Input: dimensioned drawing with shaded views. Units: mm. Origin: part minimum x, y, z. A direction names the side the tool comes from. Give positions to 0.01 mm unless a question says otherwise; leave off trailing zeros. Write each loop counter-clockwise with the first axis right and the second up, starting at its lowest first coordinate (ties: lowest second). Pieces come first, ordered by that corner, then holes. Notation, with made-up numbers: M 4.25,33 L 25.25,33 A31 cw 25.25,66 Z; hole C 40.25,77 d10. An arc over 180 degrees is marked long. Answer as a JSON object with one key per item and string values.
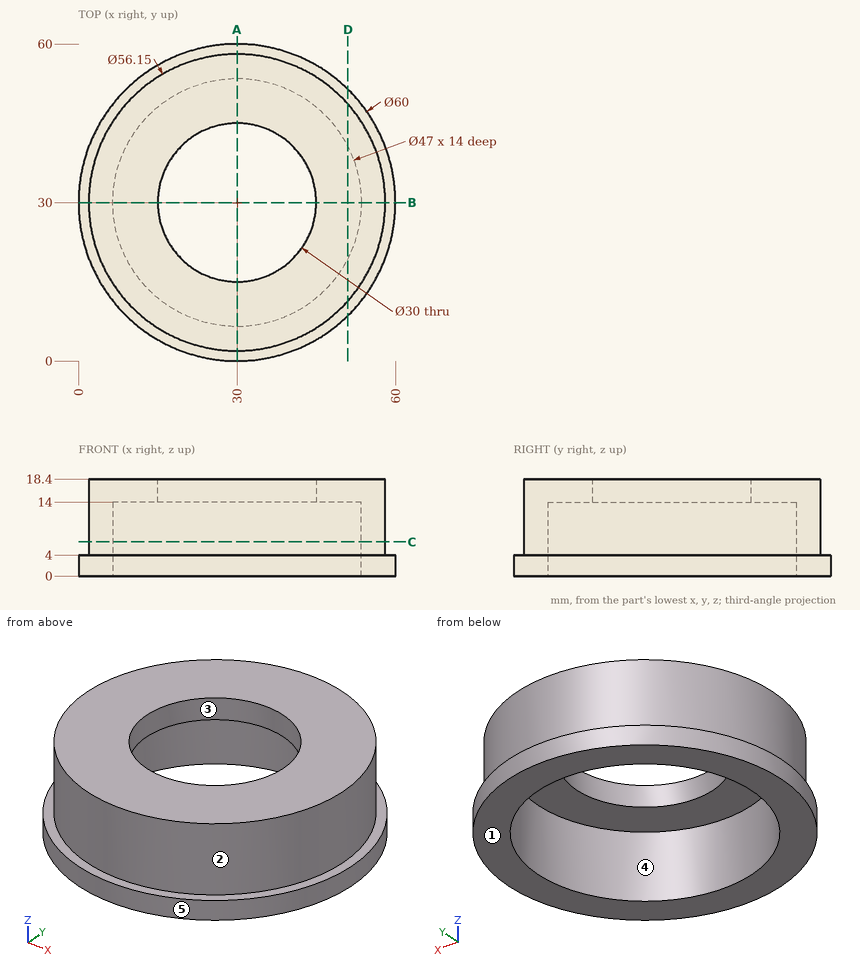
1) Line query: line 1 (Y direction, x = 30, z = 16.4) (3 decimals); line 2 (Y direction, x = 30, z = 5.75) (3 decimals); line 3 (Z direction, x = 7, y = 33.5). Output: solid intervals per line, ascending. Write a range as from..to.
Geometry check:
{"line 1": "y = 1.925..15, 45..58.075", "line 2": "y = 1.925..6.5, 53.5..58.075", "line 3": "z = 14..18.4"}
2) Cut plane D-D on x = 51. Return loops of the section in (y, z).
Geometry check:
{"outline": "M 8.58,0 L 19.45,0 L 19.45,14 L 40.55,14 L 40.55,0 L 51.42,0 L 51.42,4 L 48.63,4 L 48.63,18.4 L 11.37,18.4 L 11.37,4 L 8.58,4 Z"}
3) Cut plane A-A on x = 30. Return loops of the section in (y, z) (3 decimals), and give its area (3 significant figures).
Geometry check:
{"outline": "M 0,0 L 6.5,0 L 6.5,14 L 15,14 L 15,18.4 L 1.925,18.4 L 1.925,4 L 0,4 Z; M 45,14 L 53.5,14 L 53.5,0 L 60,0 L 60,4 L 58.075,4 L 58.075,18.4 L 45,18.4 Z", "area": "259 mm2"}
4) Set-up query: the marked faces 4 and 5. Return all of +Z, -Z, +X, -X, +Y, -Y with unobstructed straight access to the full face (end or side cutting, diameter ignored); none if empty.
Geometry check:
{"face 4": "-Z", "face 5": "+Z, -Z"}
5) Pull-direction query (X, two-part tool) for the marked faces 1, 2 and 3; classes: pulls with the +X half, pulls with the -X half, needs draft (parallel to the pull), parting line crosses it, or undercut.
Geometry check:
{"face 1": "needs draft", "face 2": "parting line crosses it", "face 3": "undercut"}
6) Contact query for flat-ended pins moving along their axis: P1, Ø3, axis at y = 27.5, z = 10, coming from the -X side; P2, Ø1.5, axis at x = 33.5, z = 5.5, coming from the -Y side; P3, Ø1.5, axis at y = 41.5, z = 14, coming from the +X side. Output: stop coordinate, or through.
Geometry check:
{"P1": "stops at x = 1.94", "P2": "stops at y = 2.06", "P3": "stops at x = 55.94"}
7) Cut plane C-C on z = 6.5. Return loops of the section in (x, y) (3 decimals).
Geometry check:
{"outline": "C 30,30 d56.15; hole C 30,30 d47"}
